from build123d import *

# Parameters (mm, degrees)
SKETCH1_W           = 52
SKETCH1_H           = 20
BOSS_EXTRUDE1_DEPTH = 25
SKETCH2_W           = 21
SKETCH2_H           = 10
CUT_EXTRUDE1_DEPTH  = 152.858008365
CUT_EXTRUDE2_DEPTH  = 542.477569293
SKETCH4_R           = 1.6
CUT_EXTRUDE3_DEPTH  = 542.477569293
SKETCH5_W           = 22
SKETCH5_H           = 10
CUT_EXTRUDE4_DEPTH  = 4
SKETCH6_R           = 1.6
CUT_EXTRUDE5_DEPTH  = 4
SKETCH7_W           = 6
SKETCH7_H           = 7
CUT_EXTRUDE6_DEPTH  = 1
SKETCH8_W           = 6
SKETCH8_H           = 7
CUT_EXTRUDE7_DEPTH  = 1
SKETCH9_R           = 3
CUT_EXTRUDE8_DEPTH  = 1


with BuildPart() as part:
    # Sketch1 → Boss-Extrude1 (new body)
    with BuildSketch(Plane.XY):
        with Locations((514.530256366, 130.470120327)):
            Rectangle(SKETCH1_W, SKETCH1_H)
    extrude(amount=BOSS_EXTRUDE1_DEPTH)

    # Sketch2 → Cut-Extrude1 (cut, through all)
    with BuildSketch(Plane(origin=(540.530256366, 0, 0), x_dir=(0, 0, -1), z_dir=(1, 0, 0))):
        with Locations((-10.5, 130.470120327)):
            Rectangle(SKETCH2_W, SKETCH2_H)
    extrude(amount=-CUT_EXTRUDE1_DEPTH, mode=Mode.SUBTRACT)

    # Sketch3 → Cut-Extrude2 (cut, through all)
    with BuildSketch(Plane(origin=(0, 140.470120327, 0), x_dir=(1, 0, 0), z_dir=(0, 1, 0))):
        Polygon((488.530256366, -19), (503.530256366, 0), (525.530256366, 0), (540.530256366, -19), (550.000331081, -19), (550.000331081, 5.4233188), (484.277494653, 5.4233188), (484.277494653, -19), align=None)
    extrude(amount=-CUT_EXTRUDE2_DEPTH, mode=Mode.SUBTRACT)

    # Sketch4 → Cut-Extrude3 (cut, through all)
    with BuildSketch(Plane(origin=(0, 140.470120327, 0), x_dir=(1, 0, 0), z_dir=(0, 1, 0))):
        with Locations(Location((514.530256366, -9, 0), (0, 0, 270))):
            Circle(SKETCH4_R)
    extrude(amount=-CUT_EXTRUDE3_DEPTH, mode=Mode.SUBTRACT)

    # Sketch5 → Cut-Extrude4 (cut)
    with BuildSketch(Plane(origin=(0, 0, 21), x_dir=(-1, 0, 0), z_dir=(0, 0, -1))):
        with Locations((-514.530256366, 130.470120327)):
            Rectangle(SKETCH5_W, SKETCH5_H)
    extrude(amount=-CUT_EXTRUDE4_DEPTH, mode=Mode.SUBTRACT)

    # Sketch6 → Cut-Extrude5 (cut)
    with BuildSketch(Plane(origin=(0, 0, 21), x_dir=(-1, 0, 0), z_dir=(0, 0, -1))):
        with Locations((-533.030256366, 130.470120327)):
            Circle(SKETCH6_R)
        with Locations((-496.030256366, 130.470120327)):
            Circle(SKETCH6_R)
    extrude(amount=-CUT_EXTRUDE5_DEPTH, mode=Mode.SUBTRACT)

    # Sketch7 → Cut-Extrude6 (cut)
    with BuildSketch(Plane(origin=(0, 0, 21), x_dir=(-1, 0, 0), z_dir=(0, 0, -1))):
        with Locations((-496.030256366, 130.470120327)):
            Rectangle(SKETCH7_W, SKETCH7_H)
    extrude(amount=-CUT_EXTRUDE6_DEPTH, mode=Mode.SUBTRACT)

    # Sketch8 → Cut-Extrude7 (cut)
    with BuildSketch(Plane(origin=(0, 0, 21), x_dir=(-1, 0, 0), z_dir=(0, 0, -1))):
        with Locations((-533.030256366, 130.470120327)):
            Rectangle(SKETCH8_W, SKETCH8_H)
    extrude(amount=-CUT_EXTRUDE7_DEPTH, mode=Mode.SUBTRACT)

    # Sketch9 → Cut-Extrude8 (cut)
    with BuildSketch(Plane(origin=(0, 140.470120327, 0), x_dir=(1, 0, 0), z_dir=(0, 1, 0))):
        with Locations(Location((514.530256366, -9, 0), (0, 0, 270))):
            Circle(SKETCH9_R)
    extrude(amount=-CUT_EXTRUDE8_DEPTH, mode=Mode.SUBTRACT)


solid = part.part
Build history of the part. All positions in model axes, mm. A direction names the side the tool comes from. Coordinates: 2 decimals unless noted, no trailing zeros. Write each loop counter-clockwise with the first axis right and the second up, starting at its lowest first coordinate (ties: lowest second). Pieces come first, ordered by that corner, then holes.
(1) Mould opens along Y. For faces 4 (the flat face through (496.1, 133.97, 21.5)), 5 (the flat face through (514, 140.47, 15)), 6 (the flat face through (540.53, 130, 23)) say: pulls with the +Y half, pulls with the -Y half, needs draft (parallel to the pull), parting line crosses it, or undercut.
(2) Cut at A-A on y = 132.75. List the corners of the cut face in (x, z), and give its area (3 significant figures).
(3) Pin check, flat tips, straight feed: pin 1 Ø5 at (x, y) = (501.5, 132.5) entering from -Z; pin 2 Ø4 at (x, y) = (496.03, 130.47) entering from -Z; pin 3 Ø12 at (x, y) = (500, 123) entering from -Z. Stop position of each tip, or through.
(4) Cut at D-D on z = 9. List the corners of the cut face in (x, y) (3 decimals).
(5) 3-axis set-ups, long thin cutter, end or side, ignore diameter. For faces 1 (the flat face through (525.53, 130, 23)), 2 (the flat face through (497, 132, 22)), 3 (the flat face through (513, 139.47, 10)): which of +Z, -Z, +X, -X, +Y, -Y reach the whole face in a straight line?
(6) Drill centre lines: line 1 (Y direction, x = 522.5, z = 23); line 2 (Z direction, x = 492.5, y = 129.75); line 3 (X direction, y = 139.8, z = 9) (3 decimals). Where is each one in solid material? Low to high.
(7) Cut at B-B on x = 524. List the corners of the cut face in (y, z).
(8) Cut at C-C on z = 20.5. List the corners of the cut face in (x, y), and give its area (3 significant figures).
Working result:
1. face 4: undercut
1. face 5: pulls with the +Y half
1. face 6: needs draft
2. outline: (488.53, 21) - (493.03, 21) - (493.03, 22) - (499.03, 22) - (499.03, 21) - (503.53, 21) - (503.53, 25) - (488.53, 25) - close; (525.53, 21) - (530.03, 21) - (530.03, 22) - (536.03, 22) - (536.03, 21) - (540.53, 21) - (540.53, 25) - (525.53, 25) - close
2. area: 108 mm2
3. pin 1: stops at z = 21
3. pin 2: stops at z = 22
3. pin 3: stops at z = 0
4. outline: (496.425, 120.47) - (512.93, 120.47) - (512.93, 125.47) - (496.425, 125.47) - close; (496.425, 135.47) - (512.93, 135.47) - (512.93, 139.47) - (511.53, 139.47) - (511.53, 140.47) - (496.425, 140.47) - close; (516.13, 120.47) - (532.636, 120.47) - (532.636, 125.47) - (516.13, 125.47) - close; (516.13, 135.47) - (532.636, 135.47) - (532.636, 140.47) - (517.53, 140.47) - (517.53, 139.47) - (516.13, 139.47) - close
5. face 1: +Z, -Z
5. face 2: -Z
5. face 3: +Y
6. line 1: y = 120.47 to 125.47, 135.47 to 140.47
6. line 2: z = 21 to 25
6. line 3: x = 496.425 to 511.53, 517.53 to 532.636
7. outline: (120.47, 0) - (125.47, 0) - (125.47, 25) - (120.47, 25) - close; (135.47, 0) - (140.47, 0) - (140.47, 25) - (135.47, 25) - close
8. outline: (488.53, 120.47) - (540.53, 120.47) - (540.53, 125.47) - (488.53, 125.47) - close; (488.53, 135.47) - (540.53, 135.47) - (540.53, 140.47) - (488.53, 140.47) - close
8. area: 520 mm2
